Work out the finished part from the listing and answer in its coordinate system (mm). A direction names the side the tool comes from. Round coordinates to 2 decimals unless told otherwise and drop trailing zeros. Loops run counter-clockwise (first coordinate to the right, second up) from the corner with the lowest first, then second, coordinate; pieces in that order, holes last. Notation, with made-up numbers: (55.5, -31.5) -> (104.5, -31.5) arc R14 cw to (104.5, -6.5) -> close; hole circle Ø6 at (14, 53). An arc over 180 degrees is marked (long way). Write item = value, one per line. Start each with the question number.
```python
from build123d import *

# Parameters (mm, degrees)
SKETCH_1_W             = 365
SKETCH_1_H             = 50
EXTRUDE_1_DEPTH        = 2.5
SKETCH_2_W             = 20
SKETCH_2_H             = 24
EXTRUDE_2_DEPTH        = 70
PATTERN_LINEAR_1_COUNT = 2
PATTERN_LINEAR_1_PITCH = 60
SKETCH_4_R             = 1.6
CUT_EXTRUDE_1_DEPTH    = 366.633012733
CUT_EXTRUDE_2_REACH    = 197.336
SKETCH_5_R             = 1.6
SKETCH_5_R_2           = 10


with BuildPart() as part:
    # 草图1 → 凸台-拉伸1 (new, symmetric)
    with BuildSketch(Plane.XY):
        Rectangle(SKETCH_1_W, SKETCH_1_H)
    extrude_1 = extrude(amount=EXTRUDE_1_DEPTH, both=True)

    # 草图2 → 凸台-拉伸2 (add)
    with BuildSketch(Plane.XY.offset(2.5)):
        with Locations((165, 0)):
            Rectangle(SKETCH_2_W, SKETCH_2_H)
        with Locations((-165, 0)):
            Rectangle(SKETCH_2_W, SKETCH_2_H)
    extrude(amount=EXTRUDE_2_DEPTH)

    # 阵列(线性)1: 凸台-拉伸1 ×2
    with Locations(*[(0, 0, i * PATTERN_LINEAR_1_PITCH) for i in range(1, PATTERN_LINEAR_1_COUNT)]):
        add(extrude_1)

    # 草图4 → 切除-拉伸1 (cut, through all)
    with BuildSketch(Plane.ZY.offset(175)):
        with Locations((67.5, 4.5)):
            Circle(SKETCH_4_R)
    cut_extrude_1 = extrude(amount=-CUT_EXTRUDE_1_DEPTH, mode=Mode.SUBTRACT)

    # 草图5 → 切除-拉伸2 (cut, up to next)
    with BuildSketch(Plane.XY.offset(62.5), mode=Mode.PRIVATE) as cut_extrude_2_sk1:
        with Locations((-15.5, 15.5)):
            Circle(SKETCH_5_R)
    cut_extrude_2_tool1 = extrude(cut_extrude_2_sk1.sketch, amount=-CUT_EXTRUDE_2_REACH, mode=Mode.PRIVATE) & part.part
    # 草图5 → 切除-拉伸2 (cut, up to next)
    with BuildSketch(Plane.XY.offset(62.5), mode=Mode.PRIVATE) as cut_extrude_2_sk2:
        with Locations((15.5, 15.5)):
            Circle(SKETCH_5_R)
    cut_extrude_2_tool2 = extrude(cut_extrude_2_sk2.sketch, amount=-CUT_EXTRUDE_2_REACH, mode=Mode.PRIVATE) & part.part
    # 草图5 → 切除-拉伸2 (cut, up to next)
    with BuildSketch(Plane.XY.offset(62.5), mode=Mode.PRIVATE) as cut_extrude_2_sk3:
        with Locations((15.5, -15.5)):
            Circle(SKETCH_5_R)
    cut_extrude_2_tool3 = extrude(cut_extrude_2_sk3.sketch, amount=-CUT_EXTRUDE_2_REACH, mode=Mode.PRIVATE) & part.part
    # 草图5 → 切除-拉伸2 (cut, up to next)
    with BuildSketch(Plane.XY.offset(62.5), mode=Mode.PRIVATE) as cut_extrude_2_sk4:
        with Locations((-15.5, -15.5)):
            Circle(SKETCH_5_R)
    cut_extrude_2_tool4 = extrude(cut_extrude_2_sk4.sketch, amount=-CUT_EXTRUDE_2_REACH, mode=Mode.PRIVATE) & part.part
    # 草图5 → 切除-拉伸2 (cut, up to next)
    with BuildSketch(Plane.XY.offset(62.5), mode=Mode.PRIVATE) as cut_extrude_2_sk5:
        Circle(SKETCH_5_R_2)
    cut_extrude_2_tool5 = extrude(cut_extrude_2_sk5.sketch, amount=-CUT_EXTRUDE_2_REACH, mode=Mode.PRIVATE) & part.part
    add(cut_extrude_2_tool1.solids().sort_by_distance((-15.5, 15.5, 62.5))[0], mode=Mode.SUBTRACT)
    add(cut_extrude_2_tool2.solids().sort_by_distance((15.5, 15.5, 62.5))[0], mode=Mode.SUBTRACT)
    add(cut_extrude_2_tool3.solids().sort_by_distance((15.5, -15.5, 62.5))[0], mode=Mode.SUBTRACT)
    add(cut_extrude_2_tool4.solids().sort_by_distance((-15.5, -15.5, 62.5))[0], mode=Mode.SUBTRACT)
    add(cut_extrude_2_tool5.solids().sort_by_distance((0, 0, 62.5))[0], mode=Mode.SUBTRACT)

    # 镜向1: 切除-拉伸1 across plane
    add(cut_extrude_1.mirror(Plane.ZX), mode=Mode.SUBTRACT)


solid = part.part
```
Item 1: Section C-C (x = 0) is taken. Determine the outline of the cut face in (y, z).
Item 2: Flat-ended cylindrical pins translate along their axes: pin 1 (5 mm diameter, centred on x = -166.5, z = 66.5, fed in from -Y); pin 2 (1 mm diameter, centred on y = 13, z = 24, fed in from +X); pin 3 (5 mm diameter, centred on x = -167.5, z = 67, fed in from +Y); pin 4 (11 mm diameter, centred on y = -5.5, z = 69, fed in from +X). Find the tip coordinate at first contact, or state that the pin passes through.
Item 3: Find the intervals of material crossed by line 1 along Y through (x, z) = (-164.5, 67.5); line 2 along Y through (x, z) = (-15.5, 59.1); line 3 along Z through (x, y) = (-128, 2.5), in increasing order. Write a range as [from, to].
Item 4: Section B-B (y = 21) is taken. Determine the outline of the cut face in (x, z).
Item 5: The mould has two halves that part along Y. Classify faces 5 (the cylindrical face through (-2.17, -9.76, 60.04)), 6 (the flat face through (165, -12, 67)), 7 (the flat face through (-175, 0, 30)): pulls with the +Y half, pulls with the -Y half, needs draft (parallel to the pull), parting line crosses it, or undercut.
Item 6: A tool of negligible diameter and unlimited length cuts with its end or side. For faces 1 (the flat face through (155, 0, 30)), 2 (the flat face through (175, 0, 30)), 3 (the flat face through (-155, 0, 67)), 4 (the flat face through (-165, 12, 30)), from which of +Z, -Z, +X, -X, +Y, -Y can it reach the whole face along a straight path? Write none if from no direction.
Item 7: Section A-A (z = 21.5) is taken. Determine the outline of the cut face in (x, y).
Worked answers:
q1.outline = (-25, -2.5) -> (25, -2.5) -> (25, 2.5) -> (-25, 2.5) -> close; (-25, 57.5) -> (-10, 57.5) -> (-10, 62.5) -> (-25, 62.5) -> close; (10, 57.5) -> (25, 57.5) -> (25, 62.5) -> (10, 62.5) -> close
q2.pin_1 = -12
q2.pin_2 = through
q2.pin_3 = 12
q2.pin_4 = 175
q3.line_1 = [-12, -6.1], [-2.9, 2.9], [6.1, 12]
q3.line_2 = [-25, -17.1], [-13.9, 13.9], [17.1, 25]
q3.line_3 = [-2.5, 2.5], [57.5, 62.5]
q4.outline = (-182.5, -2.5) -> (182.5, -2.5) -> (182.5, 2.5) -> (-182.5, 2.5) -> close; (-182.5, 57.5) -> (182.5, 57.5) -> (182.5, 62.5) -> (-182.5, 62.5) -> close
q5.face_5 = undercut
q5.face_6 = pulls with the -Y half
q5.face_7 = needs draft
q6.face_1 = +Y, -Y
q6.face_2 = +X, +Y, -Y
q6.face_3 = +Z, +Y, -Y
q6.face_4 = +X, -X, +Y
q7.outline = (-175, -12) -> (-155, -12) -> (-155, 12) -> (-175, 12) -> close; (155, -12) -> (175, -12) -> (175, 12) -> (155, 12) -> close
